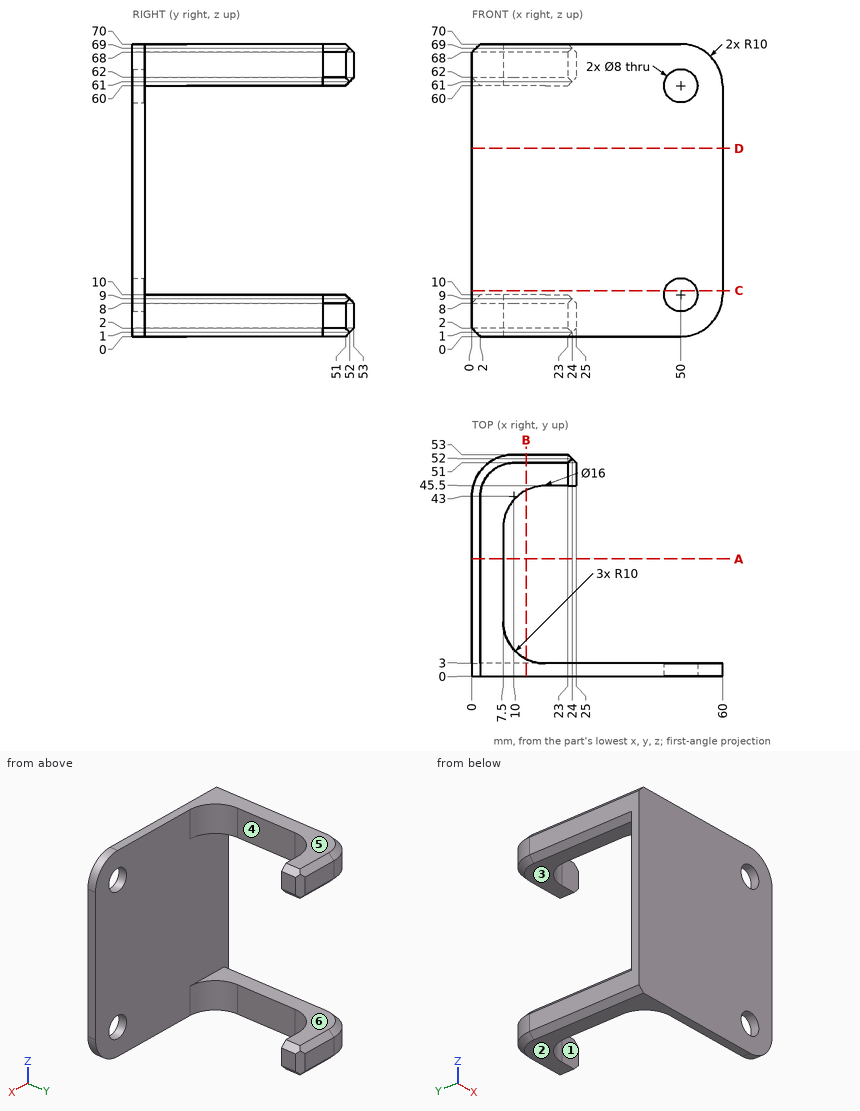
Input: dimensioned drawing with shaded views. Units: mm. Origin: part minimum x, y, z. A direction names the side the tool comes from. Give positions to 0.01 mm unless a question says otherwise; leave off trailing zeros. Write each loop counter-clockwise with the first axis right and the second up, starting at its lowest first coordinate (ties: lowest second). Pieces come first, ordered by that corner, then holes.
Q1. Section D-D, the plane z = 45. Output: boundary loops of the cut face in (x, y).
Q2. Pull-direction query (Z, two-part tool) for the marked faces 3, 4, 5 and 6; classes: pulls with the +Z half, pulls with the -Z half, needs draft (parallel to the pull), parting line crosses it, or undercut.
Q3. Section A-A, the plane y = 28. Output: boundary loops of the cut face in (x, z).
Q4. Section C-C, the plane z = 11. Output: boundary loops of the cut face in (x, y).
Q5. Set-up query: the marked faces 1 and 2. Return all of +Z, -Z, +X, -X, +Y, -Y with unobstructed straight access to the full face (end or side cutting, diameter ignored); none if empty.
Q6. First-contact query: P1, Ø11, axis at y = 29.5, z = 62.5, coming from the +X side; P2, Ø3, axis at y = 48, z = 5, coming from the +X side; P3, Ø12, axis at x = 46.5, z = 27, coming from the +Y side. Flat tips, straight axial feed; report the tip coordinate or a pass-through.
Q7. Section B-B, the plane x = 13. Output: boundary loops of the cut face in (y, z), plus the area to 3 significant figures.
Q8. Material intervals for probe 1 along Z at (x, y) = (50, 2); probe 2 along Z at (x, y) = (13, 47.5); probe 3 along X at (y, z) = (1, 60), sorted ascending.
Filled in:
1. outline: (0, 0) - (60, 0) - (60, 3) - (0, 3) - close
2. face 3: undercut
2. face 4: needs draft
2. face 5: pulls with the +Z half
2. face 6: undercut
3. outline: (0, 2) - (2, 0) - (7.5, 0) - (7.5, 10) - (2, 10) - (0, 8) - close; (0, 62) - (2, 60) - (7.5, 60) - (7.5, 70) - (2, 70) - (0, 68) - close
4. outline: (0, 0) - (46.13, 0) - (46.13, 3) - (0, 3) - close; (53.87, 0) - (60, 0) - (60, 3) - (53.87, 3) - close
5. face 1: +Z, -Z, +X
5. face 2: -Z, +X, -X, +Y, -Y
6. P1: stops at x = 7.5
6. P2: stops at x = 25
6. P3: stops at y = 3
7. outline: (0, 0) - (4.07, 0) - (4.07, 10) - (3, 10) - (3, 60) - (4.07, 60) - (4.07, 70) - (0, 70) - close; (44.43, 0) - (51, 0) - (53, 2) - (53, 8) - (51, 10) - (44.43, 10) - close; (44.43, 60) - (51, 60) - (53, 62) - (53, 68) - (51, 70) - (44.43, 70) - close
7. area: 395 mm2
8. probe 1: z = 0 to 6, 14 to 56, 64 to 70
8. probe 2: z = 0 to 10, 60 to 70
8. probe 3: x = 0 to 46, 54 to 60
